For this review, take the finished solid that the model builds, in its own axes (mm). Face numbers are marked on the shaded views. A direction names the side the tool comes from. Coordinates: 2 decimals unless noted, no trailing zeros. Write each loop counter-clockwise with the first axis right and the second up, starting at its lowest first coordinate (ties: lowest second). Pieces come first, ordered by that corner, then holes. Notation, with made-up numbers: (-34, -6.75) - (24, -6.75) arc R26 ccw to (24, 31.25) - close; hole circle Ø10 at (53, 73). An arc over 180 degrees is marked (long way). Use one line per item in the form item = value. Start each with the question number.
1) Tool access review of the marked faces 1, 2, 3 and 4: name each direction out of +Z, -Z, +X, -X, +Y, -Y from which nothing blocks a thin tool from reaching the whole face with its end or side.
2) Insertion check: P1, Ø8, axis at y = -10.5, z = 10.5, coming from the +X side; P2, Ø0.5, axis at y = 3.5, z = 11, coming from the +X side; P3, Ø12.5, axis at x = 0.5, z = 7.5, coming from the +Y side; P4, Ø9, axis at y = 1, z = 15, coming from the +X side. Each pin has a flat end and moves straight along its axis. Give the tip position at first contact, or say it passes through.
3) We need section B-B (z = 4.5). Count the separate pieces of the cut face and the enclosed holes in it, plus the area to 3 significant figures.
4) Mouldability with a two-part tool opening along Z and no side actions: class the marked faces 5, 6, 7 and 8 as pulls with the +Z half, pulls with the -Z half, needs draft (parallel to the pull), parting line crosses it, or undercut.
5) We need section A-A (x = 0). Give the boundary of the cut face in (y, z), plus the area to 3 significant figures.
6) For L1, parallel to Y at x = 3, z = 9.75; L2, parallel to X at y = -4.5, z = 4.5; L3, parallel to X at y = 1.75, z = 11.5, list the stretches that pass through material, from the lowest coordinate up. Write a range as from..to.
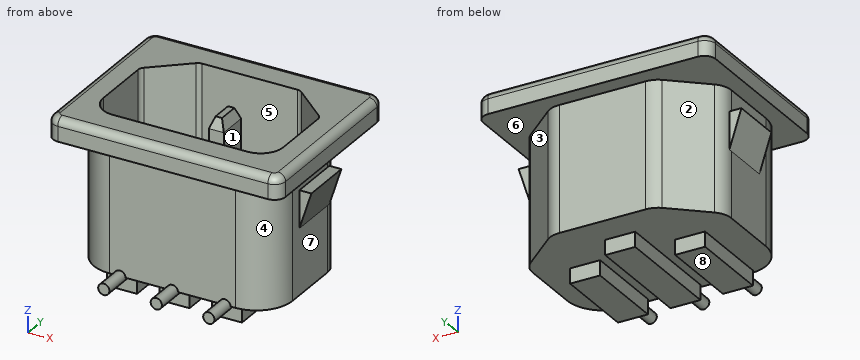
```python
from build123d import *

# Parameters (mm, degrees)
EXTRUDE1_DEPTH         = 19.75
CUT_EXTRUDE1_DEPTH     = 17
SKETCH3_OUTSIDE_W      = 41.78
SKETCH3_OUTSIDE_H      = 34.78
CUT_EXTRUDE2_DEPTH     = 16.75
SKETCH4_W              = 2
SKETCH4_H              = 4
EXTRUDE2_DEPTH         = 15
SKETCH5_W              = 2
SKETCH5_H              = 4
CUT_EXTRUDE3_DEPTH     = 3
CHAMFER1_SIZE          = 1.5
CHAMFER1_SIZE2         = 0.575796053
CHAMFER1_PART_2_SIZE   = 1.5
CHAMFER1_PART_2_SIZE2  = 0.575796053
CHAMFER1_PART_3_SIZE   = 1.5
CHAMFER1_PART_3_SIZE2  = 0.575796053
CHAMFER1_PART_4_SIZE   = 1.5
CHAMFER1_PART_4_SIZE2  = 0.575796053
CHAMFER1_PART_5_SIZE   = 1.5
CHAMFER1_PART_5_SIZE2  = 0.575796053
CHAMFER1_PART_6_SIZE   = 1.5
CHAMFER1_PART_6_SIZE2  = 0.575796053
CHAMFER1_PART_7_SIZE   = 1.5
CHAMFER1_PART_7_SIZE2  = 0.575796053
CHAMFER1_PART_8_SIZE   = 1.5
CHAMFER1_PART_8_SIZE2  = 0.575796053
CHAMFER1_PART_9_SIZE   = 1.5
CHAMFER1_PART_9_SIZE2  = 0.575796053
CHAMFER1_PART_10_SIZE  = 1.5
CHAMFER1_PART_10_SIZE2 = 0.575796053
CHAMFER1_PART_11_SIZE  = 1.5
CHAMFER1_PART_11_SIZE2 = 0.575796053
CHAMFER1_PART_12_SIZE  = 1.5
CHAMFER1_PART_12_SIZE2 = 0.575796053
FILLET1_R              = 1
EXTRUDE3_DEPTH         = 3.45
SKETCH7_W              = 4
SKETCH7_H              = 15
SKETCH7_H_2            = 11
EXTRUDE4_DEPTH         = 2
SKETCH8_R              = 0.75
EXTRUDE5_DEPTH         = 4.2


with BuildPart() as part:
    # Sketch1 → Extrude1 (new body)
    with BuildSketch(Plane.XY):
        with BuildLine():
            Line((-14, -12), (14, -12))
            ThreePointArc((14, -12), (15.060660172, -11.560660172), (15.5, -10.5))
            Line((15.5, -10.5), (15.5, 10.5))
            ThreePointArc((15.5, 10.5), (15.060660172, 11.560660172), (14, 12))
            Line((14, 12), (-14, 12))
            ThreePointArc((-14, 12), (-15.060660172, 11.560660172), (-15.5, 10.5))
            Line((-15.5, 10.5), (-15.5, -10.5))
            ThreePointArc((-15.5, -10.5), (-15.060660172, -11.560660172), (-14, -12))
        make_face()
    extrude(amount=EXTRUDE1_DEPTH)

    # Sketch2 → Cut-Extrude1 (cut)
    with BuildSketch(Plane.XY.offset(19.75)):
        with BuildLine():
            Line((-12, 3), (-12, -5))
            ThreePointArc((-12, -5), (-11.121320344, -7.121320344), (-9, -8))
            Line((-9, -8), (9, -8))
            ThreePointArc((9, -8), (11.121320344, -7.121320344), (12, -5))
            Line((12, -5), (12, 3))
            ThreePointArc((12, 3), (11.908882001, 3.417053364), (11.652132983, 3.758104592))
            Line((11.652132983, 3.758104592), (7.002132983, 7.758104592))
            ThreePointArc((7.002132983, 7.758104592), (6.697775364, 7.937577888), (6.35, 8))
            Line((6.35, 8), (-6.35, 8))
            ThreePointArc((-6.35, 8), (-6.697775364, 7.937577888), (-7.002132983, 7.758104592))
            Line((-7.002132983, 7.758104592), (-11.652132983, 3.758104592))
            ThreePointArc((-11.652132983, 3.758104592), (-11.908882001, 3.417053364), (-12, 3))
        make_face()
    extrude(amount=-CUT_EXTRUDE1_DEPTH, mode=Mode.SUBTRACT)

    # Sketch3 outside → Cut-Extrude2 (cut)
    with BuildSketch(Plane(origin=(0, 0, 0), x_dir=(-1, 0, 0), z_dir=(0, 0, -1))):
        Rectangle(SKETCH3_OUTSIDE_W, SKETCH3_OUTSIDE_H)
        with BuildLine():
            Line((13.25, 3), (13.25, -5))
            ThreePointArc((13.25, -5), (11.811910569, -8.397190887), (8.4, -9.8))
            Line((8.4, -9.8), (-8.4, -9.8))
            ThreePointArc((-8.4, -9.8), (-11.811910569, -8.397190887), (-13.25, -5))
            Line((-13.25, -5), (-13.25, 3))
            ThreePointArc((-13.25, 3), (-12.990313702, 4.188602088), (-12.258579001, 5.160598088))
            Line((-12.258579001, 5.160598088), (-7.608579001, 9.160598088))
            ThreePointArc((-7.608579001, 9.160598088), (-6.736153383, 9.645587911), (-5.75, 9.8))
            Line((-5.75, 9.8), (5.75, 9.8))
            ThreePointArc((5.75, 9.8), (6.736153383, 9.645587911), (7.608579001, 9.160598088))
            Line((7.608579001, 9.160598088), (12.258579001, 5.160598088))
            ThreePointArc((12.258579001, 5.160598088), (12.990313702, 4.188602088), (13.25, 3))
        make_face(mode=Mode.SUBTRACT)
    extrude(amount=-CUT_EXTRUDE2_DEPTH, mode=Mode.SUBTRACT)

    # Sketch4 → Extrude2 (add)
    with BuildSketch(Plane.XY.offset(2.75)):
        with Locations((0, 2.3)):
            Rectangle(SKETCH4_W, SKETCH4_H)
        with Locations((-7, -2.2)):
            Rectangle(SKETCH4_W, SKETCH4_H)
        with Locations((7, -2.2)):
            Rectangle(SKETCH4_W, SKETCH4_H)
    extrude(amount=EXTRUDE2_DEPTH)

    # Sketch5 → Cut-Extrude3 (cut)
    with BuildSketch(Plane.XY.offset(17.75)):
        with Locations((7, -2.2)):
            Rectangle(SKETCH5_W, SKETCH5_H)
        with Locations((-7, -2.2)):
            Rectangle(SKETCH5_W, SKETCH5_H)
    extrude(amount=-CUT_EXTRUDE3_DEPTH, mode=Mode.SUBTRACT)

    # Chamfer1
    chamfer1_edges = [part.edges().sort_by_distance(p)[0] for p in [
        (0, 4.3, 17.75),
    ]]
    chamfer1_side = [part.faces().sort_by_distance(p)[0] for p in [
        (0, 4.3, 10.25),
    ]]
    chamfer(chamfer1_edges, length=CHAMFER1_SIZE, length2=CHAMFER1_SIZE2, reference=chamfer1_side[0])

    # Chamfer1 part 2
    chamfer1_part_2_edges = [part.edges().sort_by_distance(p)[0] for p in [
        (-1, 2.3, 17.75),
    ]]
    chamfer1_part_2_side = [part.faces().sort_by_distance(p)[0] for p in [
        (-1, 2.3, 10.25),
    ]]
    chamfer(chamfer1_part_2_edges, length=CHAMFER1_PART_2_SIZE, length2=CHAMFER1_PART_2_SIZE2, reference=chamfer1_part_2_side[0])

    # Chamfer1 part 3
    chamfer1_part_3_edges = [part.edges().sort_by_distance(p)[0] for p in [
        (0, 0.3, 17.75),
    ]]
    chamfer1_part_3_side = [part.faces().sort_by_distance(p)[0] for p in [
        (0, 0.3, 10.25),
    ]]
    chamfer(chamfer1_part_3_edges, length=CHAMFER1_PART_3_SIZE, length2=CHAMFER1_PART_3_SIZE2, reference=chamfer1_part_3_side[0])

    # Chamfer1 part 4
    chamfer1_part_4_edges = [part.edges().sort_by_distance(p)[0] for p in [
        (1, 2.3, 17.75),
    ]]
    chamfer1_part_4_side = [part.faces().sort_by_distance(p)[0] for p in [
        (1, 2.3, 10.25),
    ]]
    chamfer(chamfer1_part_4_edges, length=CHAMFER1_PART_4_SIZE, length2=CHAMFER1_PART_4_SIZE2, reference=chamfer1_part_4_side[0])

    # Chamfer1 part 5
    chamfer1_part_5_edges = [part.edges().sort_by_distance(p)[0] for p in [
        (7, -4.2, 14.75),
    ]]
    chamfer1_part_5_side = [part.faces().sort_by_distance(p)[0] for p in [
        (7, -4.2, 8.75),
    ]]
    chamfer(chamfer1_part_5_edges, length=CHAMFER1_PART_5_SIZE, length2=CHAMFER1_PART_5_SIZE2, reference=chamfer1_part_5_side[0])

    # Chamfer1 part 6
    chamfer1_part_6_edges = [part.edges().sort_by_distance(p)[0] for p in [
        (6, -2.2, 14.75),
    ]]
    chamfer1_part_6_side = [part.faces().sort_by_distance(p)[0] for p in [
        (6, -2.2, 8.75),
    ]]
    chamfer(chamfer1_part_6_edges, length=CHAMFER1_PART_6_SIZE, length2=CHAMFER1_PART_6_SIZE2, reference=chamfer1_part_6_side[0])

    # Chamfer1 part 7
    chamfer1_part_7_edges = [part.edges().sort_by_distance(p)[0] for p in [
        (7, -0.2, 14.75),
    ]]
    chamfer1_part_7_side = [part.faces().sort_by_distance(p)[0] for p in [
        (7, -0.2, 8.75),
    ]]
    chamfer(chamfer1_part_7_edges, length=CHAMFER1_PART_7_SIZE, length2=CHAMFER1_PART_7_SIZE2, reference=chamfer1_part_7_side[0])

    # Chamfer1 part 8
    chamfer1_part_8_edges = [part.edges().sort_by_distance(p)[0] for p in [
        (8, -2.2, 14.75),
    ]]
    chamfer1_part_8_side = [part.faces().sort_by_distance(p)[0] for p in [
        (8, -2.2, 8.75),
    ]]
    chamfer(chamfer1_part_8_edges, length=CHAMFER1_PART_8_SIZE, length2=CHAMFER1_PART_8_SIZE2, reference=chamfer1_part_8_side[0])

    # Chamfer1 part 9
    chamfer1_part_9_edges = [part.edges().sort_by_distance(p)[0] for p in [
        (-7, -4.2, 14.75),
    ]]
    chamfer1_part_9_side = [part.faces().sort_by_distance(p)[0] for p in [
        (-7, -4.2, 8.75),
    ]]
    chamfer(chamfer1_part_9_edges, length=CHAMFER1_PART_9_SIZE, length2=CHAMFER1_PART_9_SIZE2, reference=chamfer1_part_9_side[0])

    # Chamfer1 part 10
    chamfer1_part_10_edges = [part.edges().sort_by_distance(p)[0] for p in [
        (-8, -2.2, 14.75),
    ]]
    chamfer1_part_10_side = [part.faces().sort_by_distance(p)[0] for p in [
        (-8, -2.2, 8.75),
    ]]
    chamfer(chamfer1_part_10_edges, length=CHAMFER1_PART_10_SIZE, length2=CHAMFER1_PART_10_SIZE2, reference=chamfer1_part_10_side[0])

    # Chamfer1 part 11
    chamfer1_part_11_edges = [part.edges().sort_by_distance(p)[0] for p in [
        (-7, -0.2, 14.75),
    ]]
    chamfer1_part_11_side = [part.faces().sort_by_distance(p)[0] for p in [
        (-7, -0.2, 8.75),
    ]]
    chamfer(chamfer1_part_11_edges, length=CHAMFER1_PART_11_SIZE, length2=CHAMFER1_PART_11_SIZE2, reference=chamfer1_part_11_side[0])

    # Chamfer1 part 12
    chamfer1_part_12_edges = [part.edges().sort_by_distance(p)[0] for p in [
        (-6, -2.2, 14.75),
    ]]
    chamfer1_part_12_side = [part.faces().sort_by_distance(p)[0] for p in [
        (-6, -2.2, 8.75),
    ]]
    chamfer(chamfer1_part_12_edges, length=CHAMFER1_PART_12_SIZE, length2=CHAMFER1_PART_12_SIZE2, reference=chamfer1_part_12_side[0])

    # Fillet1
    fillet1_edges = [part.edges().sort_by_distance(p)[0] for p in [
        (-15.060660172, -11.560660172, 19.75),
        (0, -12, 19.75),
        (15.060660172, -11.560660172, 19.75),
        (15.5, 0, 19.75),
        (15.060660172, 11.560660172, 19.75),
        (0, 12, 19.75),
        (-15.060660172, 11.560660172, 19.75),
        (-15.5, 0, 19.75),
    ]]
    fillet(fillet1_edges, radius=FILLET1_R)

    # Sketch6 → Extrude3 (add, symmetric)
    with BuildSketch(Plane(origin=(0, 0, 0), x_dir=(1, 0, 0), z_dir=(0, 1, 0))):
        Polygon((13.25, -13.75), (13.25, -8.75), (14.85, -13.75), align=None)
        Polygon((-14.85, -13.75), (-13.25, -8.75), (-13.25, -13.75), align=None)
    extrude(amount=EXTRUDE3_DEPTH, both=True)

    # Sketch7 → Extrude4 (add)
    with BuildSketch(Plane(origin=(0, 0, 0), x_dir=(-1, 0, 0), z_dir=(0, 0, -1))):
        with Locations((0, -1.8)):
            Rectangle(SKETCH7_W, SKETCH7_H)
        with Locations((-7, -3.8)):
            Rectangle(SKETCH7_W, SKETCH7_H_2)
        with Locations((7, -3.8)):
            Rectangle(SKETCH7_W, SKETCH7_H_2)
    extrude(amount=EXTRUDE4_DEPTH)

    # Sketch8 → Extrude5 (add)
    with BuildSketch(Plane.XZ.offset(9.3)):
        with Locations((7, 0)):
            Circle(SKETCH8_R)
        Circle(SKETCH8_R)
        with Locations((-7, 0)):
            Circle(SKETCH8_R)
    extrude(amount=EXTRUDE5_DEPTH)


solid = part.part
```
Determined:
q1.face_1 = +Z
q1.face_2 = -Z, -X, +Y
q1.face_3 = -Z, +X, +Y
q1.face_4 = -Z, +X, -Y
q2.P1 = 13
q2.P2 = 14.05
q2.P3 = 9.8
q2.P4 = 15.5
q3.separate_pieces = 4
q3.enclosed_holes = 1
q3.area = 141 mm²
q4.face_5 = needs draft
q4.face_6 = undercut
q4.face_7 = undercut
q4.face_8 = pulls with the -Z half
q5.outline = (-13.5, -0.75) - (-9.3, -0.75) - (-9.3, -2) - (5.7, -2) - (5.7, 0) - (9.8, 0) - (9.8, 16.75) - (12, 16.75) - (12, 18.75) arc R1 ccw to (11, 19.75) - (8, 19.75) - (8, 2.75) - (4.3, 2.75) - (4.3, 16.25) - (3.72, 17.75) - (0.88, 17.75) - (0.3, 16.25) - (0.3, 2.75) - (-8, 2.75) - (-8, 19.75) - (-11, 19.75) arc R1 ccw to (-12, 18.75) - (-12, 16.75) - (-9.8, 16.75) - (-9.8, 0.75) - (-13.5, 0.75) - close
q5.area = 223 mm²
q6.L1 = -9.8..-8, 8..9.8
q6.L2 = -13.25..-12, 12..13.25
q6.L3 = -14.13..-12, -1..1, 12..14.13
